Work out the finished part from the listing and answer in its coordinate system (mm). A direction names the side the tool comes from. Round coordinates to 2 decimals unless told otherwise and drop trailing zeros. Write each loop counter-clockwise with the first axis right and the second up, starting at its lowest first coordinate (ties: lowest second). Pieces come first, ordered by that corner, then holes.
1. Straight lines are drawn through the part: probe 1 along Y at (x, z) = (-4.5, 2.25); probe 2 along Y at (x, z) = (0, 2.35); probe 3 along Y at (x, z) = (0, 3.6). For each, find the intervals that lie inside material, in ascending order.
2. A tool of negligible diameter and unlimited length cuts with its end or side. For faces 1 (the face through (-9, 2, 3)), 2 (the face through (-2.08, -9.366, 11.074)), 3 (the face through (8, -4, 15.3)), 4 (the face through (0, 12, 0)), 5 (the face through (9.665, 0.421, 4.564)), from which of +Z, -Z, +X, -X, +Y, -Y can it reach the whole face along a straight path? Write none if from no direction.
3. Find section A-A (z = 9.5). Write down the section's boundary in (x, y), and give its area (3 significant figures).
4. Flat-ended cylindrical pins translate along their axes: pin 1 Ø1.5 at (x, z) = (6, 4.5) entering from +Y; pin 2 Ø4 at (x, y) = (5, 0) entering from +Z; pin 3 Ø2 at (x, y) = (-11, 0) entering from +Z. Find the tip coordinate at first contact, or state that the pin passes through.
5. Determine the mould class of faces 6 (the face through (-4, -2, 2.2)), 7 (the face through (-11, -1, 3.8)), 8 (the face through (6.14, -11.8, 2.32)) for opening direction Z: pulls with the +Z half, pulls with the -Z half, needs draft (parallel to the pull), parting line crosses it, or undercut.
```python
from build123d import *

# Parameters (mm, degrees)
SKETCH1_R           = 13.3
SKETCH1_R_2         = 12.1
BOSS_EXTRUDE1_DEPTH = 3
SKETCH2_R           = 13.3
BOSS_EXTRUDE2_DEPTH = 2
SKETCH3_R           = 4
CUT_EXTRUDE1_DEPTH  = 10.2
SKETCH4_R           = 9.7
SKETCH4_R_2         = 8.5
BOSS_EXTRUDE3_DEPTH = 10.3
BOSS_EXTRUDE3_DRAFT = 1
FILLET1_R           = 2
SKETCH5_R           = 9
SKETCH5_R_2         = 4
BOSS_EXTRUDE4_DEPTH = 0.8
BOSS_EXTRUDE4_DRAFT = 1
BOSS_EXTRUDE5_DEPTH = 3
FILLET2_R           = 0.1
SKETCH7_W           = 6
SKETCH7_H           = 2
CUT_EXTRUDE2_DEPTH  = 20.8
CUT_EXTRUDE2_DRAFT  = -1
SKETCH8_R           = 0.7
CUT_EXTRUDE3_DEPTH  = 20.8
CUT_EXTRUDE4_START  = -0.8
SKETCH9_R           = 1.4
SKETCH9_R_2         = 1.5
CUT_EXTRUDE4_DEPTH  = 2
FILLET3_R           = 0.3


with BuildPart() as part:
    # Sketch1 → Boss-Extrude1 (new body)
    with BuildSketch(Plane.XY):
        Circle(SKETCH1_R)
        Circle(SKETCH1_R_2, mode=Mode.SUBTRACT)
    extrude(amount=BOSS_EXTRUDE1_DEPTH)

    # Sketch2 → Boss-Extrude2 (add)
    with BuildSketch(Plane.XY.offset(3)):
        Circle(SKETCH2_R)
    extrude(amount=BOSS_EXTRUDE2_DEPTH)

    # Sketch3 → Cut-Extrude1 (cut)
    with BuildSketch(Plane.XY.offset(5)):
        Circle(SKETCH3_R)
    extrude(amount=-CUT_EXTRUDE1_DEPTH, mode=Mode.SUBTRACT)


with BuildPart() as boss_extrude3_tool:
    # Sketch4 → Boss-Extrude3 (with draft: the straight prism first)
    with BuildSketch(Plane.XY.offset(5)):
        Circle(SKETCH4_R)
        Circle(SKETCH4_R_2, mode=Mode.SUBTRACT)
    extrude(amount=BOSS_EXTRUDE3_DEPTH)
    # Boss-Extrude3: the draft: its side faces are tilted about the plane it starts from
    boss_extrude3_sides = [boss_extrude3_tool.faces().sort_by_distance(p)[0] for p in [
        (-9.7, 0, 10.15),
        (-8.5, 0, 10.15),
    ]]
    draft(boss_extrude3_sides, Plane.XY.offset(5), BOSS_EXTRUDE3_DRAFT)


with BuildPart() as part_1:
    add(part.part)

    # Boss-Extrude3: add boss_extrude3_tool
    add(boss_extrude3_tool.part)

    # Fillet1
    fillet1_edges = [part_1.edges().sort_by_distance(p)[0] for p in [
        (-9.7, 0, 5),
    ]]
    fillet(fillet1_edges, radius=FILLET1_R)


with BuildPart() as boss_extrude4_tool:
    # Sketch5 → Boss-Extrude4 (with draft: the straight prism first)
    with BuildSketch(Plane(origin=(0, 0, 3), x_dir=(-1, 0, 0), z_dir=(0, 0, -1))):
        Circle(SKETCH5_R)
        with Locations(Location((0, 0, 0), (0, 0, 180))):
            Circle(SKETCH5_R_2, mode=Mode.SUBTRACT)
    extrude(amount=BOSS_EXTRUDE4_DEPTH)
    # Boss-Extrude4: the draft: its side faces are tilted about the plane it starts from
    boss_extrude4_sides = [boss_extrude4_tool.faces().sort_by_distance(p)[0] for p in [
        (9, 0, 2.6),
        (-4, 0, 2.6),
    ]]
    draft(boss_extrude4_sides, Plane(origin=(0, 0, 3), x_dir=(-1, 0, 0), z_dir=(0, 0, -1)), BOSS_EXTRUDE4_DRAFT)


with BuildPart() as part_2:
    add(part_1.part)

    # Boss-Extrude4: add boss_extrude4_tool
    add(boss_extrude4_tool.part)

    # Sketch6 → Boss-Extrude5 (add)
    with BuildSketch(Plane(origin=(0, 0, 0), x_dir=(-1, 0, 0), z_dir=(0, 0, -1))):
        with BuildLine():
            Line((3.029598049, 11.714586449), (2.804256045, 10.843253572))
            ThreePointArc((2.804256045, 10.843253572), (0, 11.2), (-2.804256045, 10.843253572))
            Line((-2.804256045, 10.843253572), (-3.029598049, 11.714586449))
            ThreePointArc((-3.029598049, 11.714586449), (0, 12.1), (3.029598049, 11.714586449))
        make_face()
    extrude(amount=-BOSS_EXTRUDE5_DEPTH)

    # Fillet2
    fillet2_edges = [part_2.edges().sort_by_distance(p)[0] for p in [
        (-3.029598049, 11.714586449, 1.5),
        (3.029598049, 11.714586449, 1.5),
        (2.804256045, 10.843253572, 1.5),
        (-2.804256045, 10.843253572, 1.5),
    ]]
    fillet(fillet2_edges, radius=FILLET2_R)


with BuildPart() as cut_extrude2_tool:
    # Sketch7 → Cut-Extrude2 (with draft: the straight prism first)
    with BuildSketch(Plane(origin=(0, 0, 0), x_dir=(1, 0, 0), z_dir=(0, 1, 0))):
        with Locations((0, -6.5)):
            Rectangle(SKETCH7_W, SKETCH7_H)
    extrude(amount=CUT_EXTRUDE2_DEPTH)
    # Cut-Extrude2: the draft: its side faces are tilted about the plane it starts from
    cut_extrude2_sides = [cut_extrude2_tool.faces().sort_by_distance(p)[0] for p in [
        (0, 10.4, 7.5),
        (3, 10.4, 6.5),
        (0, 10.4, 5.5),
        (-3, 10.4, 6.5),
    ]]
    draft(cut_extrude2_sides, Plane(origin=(0, 0, 0), x_dir=(1, 0, 0), z_dir=(0, 1, 0)), CUT_EXTRUDE2_DRAFT)


with BuildPart() as part_3:
    add(part_2.part)

    # Cut-Extrude2: cut by cut_extrude2_tool
    add(cut_extrude2_tool.part, mode=Mode.SUBTRACT)

    # Sketch8 → Cut-Extrude3 (cut)
    with BuildSketch(Plane(origin=(0, 0, 3), x_dir=(-1, 0, 0), z_dir=(0, 0, -1))):
        with Locations((-11, 0)):
            Circle(SKETCH8_R)
        with Locations(Location((11, 0, 0), (0, 0, 341.351023891))):
            Circle(SKETCH8_R)
    extrude(amount=-CUT_EXTRUDE3_DEPTH, mode=Mode.SUBTRACT)

    # Sketch9 → Cut-Extrude4 (cut)
    with BuildSketch(Plane(origin=(0, 0, 3), x_dir=(-1, 0, 0), z_dir=(0, 0, -1)).offset(CUT_EXTRUDE4_START)):
        with Locations((-11, 0)):
            Circle(SKETCH9_R)
        with Locations((11, 0)):
            Circle(SKETCH9_R_2)
    extrude(amount=-CUT_EXTRUDE4_DEPTH, mode=Mode.SUBTRACT)

    # Fillet3
    fillet3_edges = [part_3.edges().sort_by_distance(p)[0] for p in [
        (-13.3, 0, 5),
    ]]
    fillet(fillet3_edges, radius=FILLET3_R)


solid = part_3.part
```
Worked answers:
1. probe 1: y = -12.52 to -11.23, -7.78 to 7.78, 11.23 to 12.52
1. probe 2: y = -13.3 to -12.1, -8.99 to -4.01, 4.01 to 8.99, 11.2 to 13.3
1. probe 3: y = -13.3 to -4, 4 to 13.3
2. face 1: -Z
2. face 2: +Z
2. face 3: +Z, +X, -X, +Y, -Y
2. face 4: -Z, +X, -X, +Y, -Y
2. face 5: none
3. outline: circle Ø19.24 at (0, 0); hole circle Ø17.16 at (0, 0)
3. area: 59.6 mm2
4. pin 1: stops at y = 12.22
4. pin 2: stops at z = 5
4. pin 3: stops at z = 5.89
5. face 6: pulls with the -Z half
5. face 7: undercut
5. face 8: needs draft
